The figure shows three views and two pictorial views of one solid part (mm, origin at its lowest corner). Answer the questions. A direction names the side the tool comes from. Coordinates: 2 decimals unless noted, no trailing zeros. Order: outer loops, then holes, each group sorted by start corner. A loop starts at its lowest first (then second) coordinate and runs counter-clockwise, first axis right, second up. Notation, with made-up numbers: (71.25, -13.75) - (107.25, -13.75) arc R14 ccw to (107.25, 10.25) - close; hole circle Ø10 at (85.25, 22). An arc over 180 degrees is marked (long way). Answer as a JSON object with one key per item and string values. Group by question number.
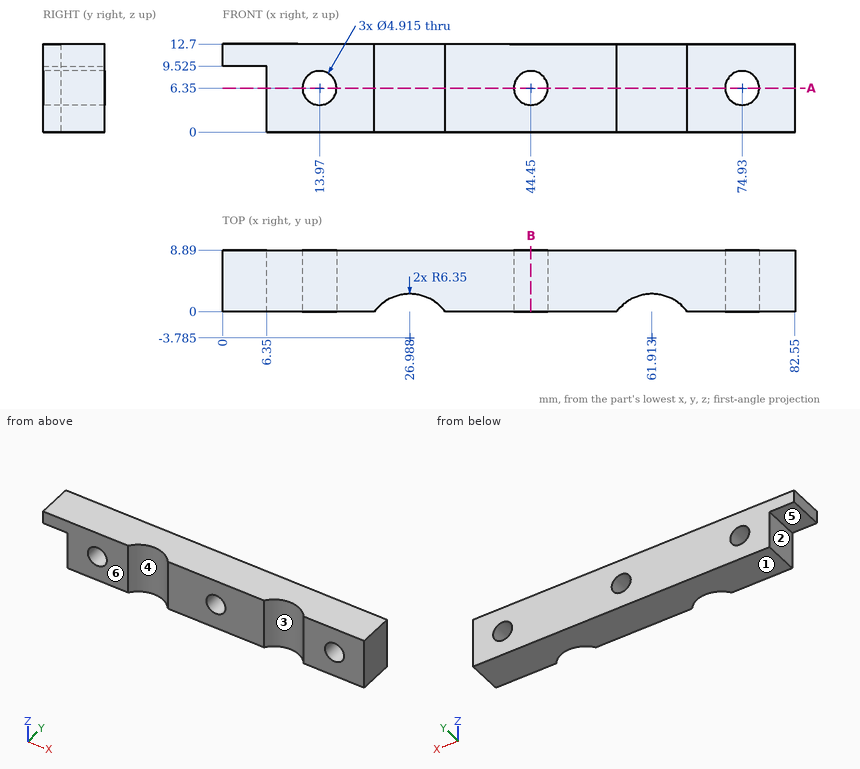
1. A cutting plane is placed at B-B on x = 44.45. Write down the section's boundary in (y, z).
2. Given pin 1 (5.5 mm diameter, centred on x = 13.97, z = 6.35, fed in from -Y); pin 2 (1.5 mm diameter, centred on y = 2.5, z = 8.5, fed in from -X); pin 3 (5 mm diameter, centred on x = 1.5, y = 3.5, fed in from -Z) (1 decimal), each flat-ended and moving along its own axis, determine where each tip first touches the part or whether it passes through.
3. For a pull along X with two mould halves and no side action, classify the marked faces 1, 2, 3 and 4 as pulls with the +X half, pulls with the -X half, needs draft (parallel to the pull), parting line crosses it, or undercut.
4. A cutting plane is placed at A-A on z = 6.35. State how many separate pieces and enclosed holes the cut face has, and give its area (3 significant figures).
5. For the marked faces 5 and 6, determine the directions among +Z, -Z, +X, -X, +Y, -Y from which every point of the face is accessible in a straight line to the end or side of a thin tool.
6. Straight lines are drawn through the part: L1, parallel to X at y = 5.25, z = 6.35; L2, parallel to X at y = 4.75, z = 7.75; L3, parallel to Z at x = 13, y = 3.25. For each, find the intervals that lie inside material, in ascending order.
Derived:
{
 "1": {"outline": "(0, 0) - (8.89, 0) - (8.89, 3.89) - (0, 3.89) - close; (0, 8.81) - (8.89, 8.81) - (8.89, 12.7) - (0, 12.7) - close"},
 "2": {"pin 1": "stops at y = 0", "pin 2": "stops at x = 6.35", "pin 3": "stops at z = 9.5"},
 "3": {"face 1": "needs draft", "face 2": "pulls with the -X half", "face 3": "undercut", "face 4": "undercut"},
 "4": {"separate pieces": "4", "enclosed holes": "0", "area": "510 mm2"},
 "5": {"face 5": "-Z, -X, +Y, -Y", "face 6": "+Z, -Z, +X, -X, -Y"},
 "6": {"L1": "x = 6.35 to 11.51, 16.43 to 41.99, 46.91 to 72.47, 77.39 to 82.55", "L2": "x = 6.35 to 11.95, 15.99 to 42.43, 46.47 to 72.91, 76.95 to 82.55", "L3": "z = 0 to 4.09, 8.61 to 12.7"}
}
